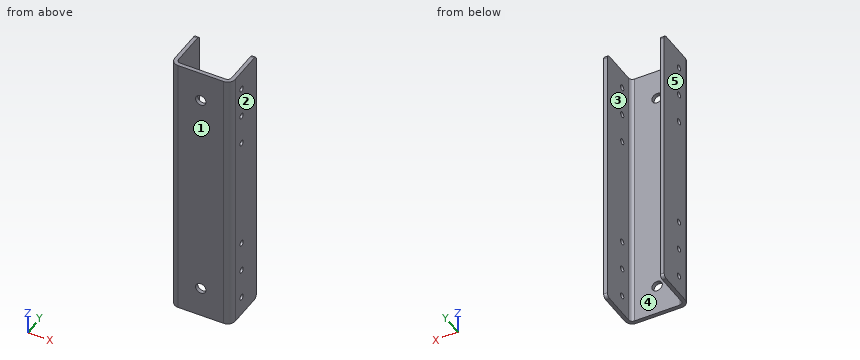
```python
from build123d import *

# Parameters (mm, degrees)
BASE_FLANGE1_DEPTH = 227.838
SKETCH6_R          = 2.4257
CUT_EXTRUDE1_DEPTH = 237.521466772
SKETCH7_R          = 4.3688
CUT_EXTRUDE2_DEPTH = 237.521466772
FILLET1_R          = 3.175


# Sheet-metal steps are written as plain solids
with BuildPart() as part:
    # Sketch1 → Base-Flange1 (new body)
    with BuildSketch(Plane.XY):
        with BuildLine():
            Line((50.8, 38.1), (50.8, 6.35))
            ThreePointArc((50.8, 6.35), (48.940128061, 1.859871939), (44.45, 0))
            Line((44.45, 0), (6.35, 0))
            ThreePointArc((6.35, 0), (1.859871939, 1.859871939), (0, 6.35))
            Line((0, 6.35), (0, 38.1))
            Line((0, 38.1), (3.175, 38.1))
            Line((3.175, 38.1), (3.175, 6.35))
            ThreePointArc((3.175, 6.35), (4.10493597, 4.10493597), (6.35, 3.175))
            Line((6.35, 3.175), (44.45, 3.175))
            ThreePointArc((44.45, 3.175), (46.69506403, 4.10493597), (47.625, 6.35))
            Line((47.625, 6.35), (47.625, 38.1))
            Line((47.625, 38.1), (50.8, 38.1))
        make_face()
    extrude(amount=BASE_FLANGE1_DEPTH)

    # Sketch6 → Cut-Extrude1 (cut, through all)
    with BuildSketch(Plane(origin=(50.8, 0, 0), x_dir=(0, 0, -1), z_dir=(1, 0, 0))):
        with Locations((-15.875, 15.875)):
            Circle(SKETCH6_R)
        with Locations((-41.275, 15.875)):
            Circle(SKETCH6_R)
        with Locations((-66.675, 15.875)):
            Circle(SKETCH6_R)
        with Locations((-161.163, 15.875)):
            Circle(SKETCH6_R)
        with Locations((-186.563, 15.875)):
            Circle(SKETCH6_R)
        with Locations((-211.963, 15.875)):
            Circle(SKETCH6_R)
    extrude(amount=-CUT_EXTRUDE1_DEPTH, mode=Mode.SUBTRACT)

    # Sketch7 → Cut-Extrude2 (cut, through all)
    with BuildSketch(Plane.XZ):
        with Locations(Location((25.4, 25.4, 0), (0, 0, 270))):
            Circle(SKETCH7_R)
        with Locations(Location((25.4, 202.438, 0), (0, 0, 270))):
            Circle(SKETCH7_R)
    extrude(amount=-CUT_EXTRUDE2_DEPTH, mode=Mode.SUBTRACT)

    # Fillet1
    fillet1_edges = [part.edges().sort_by_distance(p)[0] for p in [
        (1.5875, 38.1, 0),
        (49.2125, 38.1, 0),
        (1.5875, 38.1, 227.838),
        (49.2125, 38.1, 227.838),
    ]]
    fillet(fillet1_edges, radius=FILLET1_R)


solid = part.part
```
Here's how the part is built. I have some questions about the finished solid (model axes, mm). Face numbers are marked on the shaded views. A direction names the side the tool comes from. Coordinates: 2 decimals unless noted, no trailing zeros. Order: outer loops, then holes, each group sorted by start corner. A loop starts at its lowest first (then second) coordinate and runs counter-clockwise, first axis right, second up.
1) Imagine slicing it at C-C on x = 25.4. List the corners of the cut face in (y, z) for me (3 decimals).
2) Will these pins go through, and if not, where does the flat tip stop? pin 1 (4.5 mm diameter, centred on y = 15.875, z = 66.675, fed in from +X); pin 2 (4 mm diameter, centred on y = 4, z = 72, fed in from -X); pin 3 (3 mm diameter, centred on x = 11, z = 74, fed in from +Y) (3 decimals).
3) Imagine slicing it at D-D on x = 34. List the corners of the cut face in (y, z) for me (3 decimals), and give its area (3 significant figures).
4) Which directions (+Z, -Z, +X, -X, +Y, -Y) give clear straight access to the entire face, cutting with the end or side of a thin tool? Please do the marked faces 4 and 5.
5) I need wall thicknesses on line 1 (X direction, y = 22, z = 203.5) (3 decimals); line 2 (Y direction, x = 13.5, z = 37.5) (3 decimals); line 3 (X direction, y = 4, z = 93.5). Which ranges of each line are inside material? Lowest first, please.
6) We'd pull the mould along X, two halves only. Please class the marked faces 1, 2 and 3: +X half, -X half, draft (parallel to the pull), parting line (faces both ways), or undercut.
7) Imagine slicing it at A-A on y = 20.5. List the corners of the cut face in (x, z) for me (3 decimals).
8) Imagine slicing it at B-B on z = 25.4. List the corners of the cut face in (x, y) for me (3 decimals), and give its area (3 significant figures).
Response values:
1. outline: (0, 0) - (3.175, 0) - (3.175, 21.031) - (0, 21.031) - close; (0, 29.769) - (3.175, 29.769) - (3.175, 198.069) - (0, 198.069) - close; (0, 206.807) - (3.175, 206.807) - (3.175, 227.838) - (0, 227.838) - close
2. pin 1: passes through
2. pin 2: stops at x = 0.01
2. pin 3: stops at y = 3.175
3. outline: (0, 0) - (3.175, 0) - (3.175, 227.838) - (0, 227.838) - close
3. area: 723 mm2
4. face 4: +Z, -Z, +Y
4. face 5: +Z, -Z, -X, +Y, -Y
5. line 1: x = 0 to 3.175, 47.625 to 50.8
5. line 2: y = 0 to 3.175
5. line 3: x = 0.45 to 4.22, 46.58 to 50.35
6. face 1: draft
6. face 2: +X half
6. face 3: undercut
7. outline: (0, 0) - (3.175, 0) - (3.175, 227.838) - (0, 227.838) - close; (47.625, 0) - (50.8, 0) - (50.8, 227.838) - (47.625, 227.838) - close
8. outline: (0, 6.35) arc R6.35 ccw to (6.35, 0) - (21.031, 0) - (21.031, 3.175) - (6.35, 3.175) arc R3.175 cw to (3.175, 6.35) - (3.175, 38.1) - (0, 38.1) - close; (29.769, 0) - (44.45, 0) arc R6.35 ccw to (50.8, 6.35) - (50.8, 38.1) - (47.625, 38.1) - (47.625, 6.35) arc R3.175 cw to (44.45, 3.175) - (29.769, 3.175) - close
8. area: 342 mm2
